Can you work these out from the model? Positions are in its coordinate system, mm. Round coordinates to 2 decimals unless told otherwise and drop trailing zeros. Order: outer loops, then holes, each group sorted by start corner. A loop starts at its lowest first (then second) coordinate and runs counter-clockwise, first axis right, second up.
Q1. If we section it at A-A (x = 2.54): Please give me the cut outline in (y, z) (3 decimals), plus the area to 3 significant figures.
Q2. If we section it at C-C (y = 101.6): Please give me the cut outline in (x, z).
Q3. If we section it at B-B (y = 8.89): Please give me the cut outline in (x, z) (3 decimals).
Q4. If I drill on line 1 (X direction, y = 101.6, z = 0.65); line 2 (Y direction, x = 101.6, z = 0.8) (3 decimals); line 3 (X direction, y = 3.81, z = 0.95), over which ranges is the centre line in solid material (lowest first)?
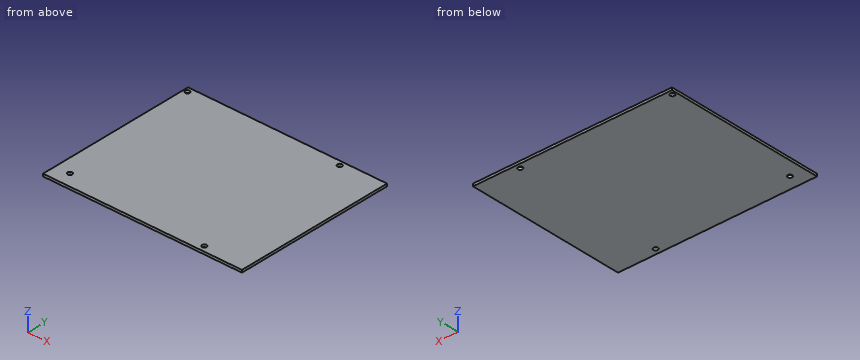
Autodesk Inventor part; units mm, degrees
ref_plane "YZ Plane" through (0, 0, 0) normal (1, 0, 0) x (0, 1, 0)
ref_plane "XZ Plane" through (0, 0, 0) normal (0, 1, 0) x (-1, 0, 0)
ref_plane "XY Plane" through (0, 0, 0) normal (0, 0, 1) x (1, 0, 0)
sketch "Sketch1" plane through (0, 0, 0) normal (0, 0, 1) x (1, 0, 0)
  line L0 (0, 0) -> (129.54, 0)
  line L1 (129.54, 0) -> (129.54, 104.775)
  line L2 (129.54, 104.775) -> (0, 104.775)
  line L3 (0, 104.775) -> (0, 0)
  dimension "d0" = 129.54
  dimension "d1" = 104.775
extrude "Extrusion1" add sketch "Sketch1" along normal blind 1.6
sketch "Sketch2" plane through (0, 0, 1.6) normal (0, 0, 1) x (1, 0, 0)
  line L0 (0, 0) -> (129.54, 0)
  line L1 (0, 104.775) -> (0, 0)
  point P0 (9.525, 8.89)
  point P1 (101.6, 3.81)
  point P2 (2.54, 101.6)
  point P3 (101.6, 101.6)
  dimension "d5" = 8.89
  dimension "d6" = 9.525
  dimension "d7" = 3.81
  dimension "d8" = 101.6
  dimension "d9" = 2.54
  dimension "d10" = 101.6
hole "Hole1" at (9.525, 8.89, 1.6) at (101.6, 3.81, 1.6) at (2.54, 101.6, 1.6) at (101.6, 101.6, 1.6) direction (0, 0, -1) diameter 3 end through all
properties part number "Smoothieboard"
Solution:
1. outline: (0, 0) - (100.1, 0) - (100.1, 1.6) - (0, 1.6) - close; (103.1, 0) - (104.775, 0) - (104.775, 1.6) - (103.1, 1.6) - close
1. area: 163 mm2
2. outline: (0, 0) - (1.04, 0) - (1.04, 1.6) - (0, 1.6) - close; (4.04, 0) - (100.1, 0) - (100.1, 1.6) - (4.04, 1.6) - close; (103.1, 0) - (129.54, 0) - (129.54, 1.6) - (103.1, 1.6) - close
3. outline: (0, 0) - (8.025, 0) - (8.025, 1.6) - (0, 1.6) - close; (11.025, 0) - (129.54, 0) - (129.54, 1.6) - (11.025, 1.6) - close
4. line 1: x = 0 to 1.04, 4.04 to 100.1, 103.1 to 129.54
4. line 2: y = 0 to 2.31, 5.31 to 100.1, 103.1 to 104.775
4. line 3: x = 0 to 100.1, 103.1 to 129.54
